The model under review builds one solid part; all positions refer to its coordinate system, in mm. A direction names the side the tool comes from. Give positions to 0.01 mm unless a question says otherwise; leave off trailing zeros. Order: outer loops, then holes, each group sorted by start corner. A loop starts at its lowest first (then second) coordinate and runs counter-clockwise, first axis right, second up. Notation, with made-up numbers: (59, 58.25) - (85, 58.25) arc R19 cw to (85, 72.25) - close; hole circle Ø7 at (70, -27.5). An arc over 180 degrees is marked (long way). Use CSV: the item, a comma, the result in double quotes.
```python
from build123d import *

# Parameters (mm, degrees)
CUT_EXTRUDE1_DEPTH = 3.5
CHAMFER1_SIZE      = 0.288675135
CHAMFER1_SIZE2     = 0.5


with BuildPart() as part:
    # Sketch1 → Revolve1 (revolve)
    with BuildSketch(Plane.XY, mode=Mode.PRIVATE) as revolve1_sk:
        Polygon((0, 0), (3, 3), (20, 3), (20, 0), align=None)
    revolve(revolve1_sk.sketch.rotate(Axis((0, 0, 0), (1, 0, 0)), 180), axis=Axis((0, 0, 0), (1, 0, 0)))

    # Sketch2 → Cut-Extrude1 (cut)
    with BuildSketch(Plane(origin=(20, 0, 0), x_dir=(0, 0, -1), z_dir=(1, 0, 0))):
        Polygon((1.732050808, 0), (0.866025404, 1.5), (-0.866025404, 1.5), (-1.732050808, 0), (-0.866025404, -1.5), (0.866025404, -1.5), align=None)
    extrude(amount=-CUT_EXTRUDE1_DEPTH, mode=Mode.SUBTRACT)

    # Chamfer1
    chamfer1_edges = [part.edges().sort_by_distance(p)[0] for p in [
        (20, 3, 0),
    ]]
    chamfer1_side = [part.faces().sort_by_distance(p)[0] for p in [
        (11.5, 3, 0),
    ]]
    chamfer(chamfer1_edges, length=CHAMFER1_SIZE, length2=CHAMFER1_SIZE2, reference=chamfer1_side[0])


solid = part.part
```
Item 1: Wall thickness on L1, parallel to Z at x = 18, y = 1.15; L2, parallel to Y at x = 9, z = 0.5; L3, parallel to Y at x = 18.75, z = -1: over which ranges is each line inside the solid? List them lowest first.
Results list:
L1,"z = -2.77 to -1.07, 1.07 to 2.77"
L2,"y = -2.96 to 2.96"
L3,"y = -2.83 to -1.27, 1.27 to 2.83"
Item 2: Tool access review of faces 1 (the face through (11.47, -2.86, -0.9)), 2 (the face through (18.274, 0.76, 1.293)): name each direction out of +Z, -Z, +X, -X, +Y, -Y from which nothing blocks a thin tool from reaching the whole face with its end or side.
Results list:
face 1,"+X, -X"
face 2,"+X"
Item 3: Take a section at A-A, the plane x = 3.5. Give the boundary of the cut face in (y, z), and give its area (3 significant figures).
Results list:
outline,"circle Ø6 at (0, 0)"
area,"28.3 mm2"
Item 4: Mouldability with a two-part tool opening along Z and no side actions: class faces 3 (the face through (20, -2, 0)), 4 (the face through (18, 1.5, 0)), 5 (the face through (1, 0, 1)) as pulls with the +Z half, pulls with the -Z half, needs draft (parallel to the pull), parting line crosses it, or undercut.
Results list:
face 3,"needs draft"
face 4,"undercut"
face 5,"parting line crosses it"
Item 5: Clearance check with a flat-ended pin moving along its axis: pin 1 (1 mm diameter, centred on x = 6.5, z = -1.5, fed in from -Y). State where the tip first meets the part, or that it passes through.
Results list:
pin 1,"stops at y = -2.83"
